For this review, take the finished solid that the model builds, in its own axes (mm). A direction names the side the tool comes from. Give positions to 0.01 mm unless a question says otherwise; leave off trailing zeros.
1) Machinability: for faces 1 (the face through (26.974, 9.148, -12.226)), 2 (the face through (129, 20, -5.5)), 3 (the face through (27.166, 88.972, -9.81)), which of the approach directions +Z, -Z, +X, -X, +Y, -Y give a long, thin tool a straight path to every point of the face, cutting with its end or side? Answer none if there is none.
2) Draft analysis for pull direction X (two halves, no side actions). For faces 4 (the face through (75, 51, 0)), 5 (the face through (0, 50, -7)), 6 (the face through (27.166, 77.722, -9.81)), state which applies: pulls with the +X half, pulls with the -X half, needs draft (parallel to the pull), parting line crosses it, or undercut.
3) For P1, Ø2.5, axis at x = 125.5, y = 9.5, coming from the +Z side; P2, Ø1.5, axis at y = 57.5, z = -12, coming from the -X side; P3, Ø3.5, axis at x = 127, y = 81.5, coming from the -Z side, all flat-tipped, find the tip position at first contact; note any pin that passes through.
4) Wall thickness on line 1 along Y through (x, z) = (127, -3.4); line 2 along Y through (x, z) = (25.5, -3.65); line 3 along Y through (x, z) = (25.5, -12): over which ranges is each line inside the solid? List them lowest first.
from build123d import *

# Parameters (mm, degrees)
F0_W           = 152.5
F0_H           = 101.5
F1_DEPTH       = 14
F2_D           = 4.2
F2_CBORE_D     = 8
F2_CBORE_DEPTH = 5.5
F4_D           = 4
F4_DEPTH       = 3.5
F4_TIP         = 1.2017212381


with BuildPart() as f1:
    # F0 (on Top) → F1 (new body)
    with BuildSketch(Plane.XY):
        with Locations((76.25, 50.75)):
            Rectangle(F0_W, F0_H)
    extrude(amount=-F1_DEPTH)

    # F2 (through all)
    with Locations(Plane.XY):
        with Locations((127, 10), (127, 21.25), (25.5, 90.25), (25.5, 79)):
            CounterBoreHole(F2_D / 2, F2_CBORE_D / 2, F2_CBORE_DEPTH)

    # F4
    with Locations(Plane(origin=(0, 0, -14), x_dir=(1, 0, 0), z_dir=(0, 0, -1))):
        with Locations((25.5, -10.5), (127, -81.5)):
            Hole(F4_D / 2, depth=F4_DEPTH)
            with Locations((0, 0, -(F4_DEPTH + F4_TIP / 2))):  # 118° drill point
                Cone(0, F4_D / 2, F4_TIP, mode=Mode.SUBTRACT)


solid = f1.part
Results list:
1. face 1: -Z
1. face 2: +Z
1. face 3: +Z, -Z
2. face 4: needs draft
2. face 5: pulls with the -X half
2. face 6: undercut
3. P1: stops at z = -5.5
3. P2: stops at x = 0
3. P3: stops at z = -10.35
4. line 1: y = 0 to 6, 14 to 17.25, 25.25 to 101.5
4. line 2: y = 0 to 75, 83 to 86.25, 94.25 to 101.5
4. line 3: y = 0 to 8.5, 12.5 to 76.9, 81.1 to 88.15, 92.35 to 101.5
